Read the model definition and answer for the solid it produces. Units are mm, in the model's axes. Face numbers are marked on the shaded views. A direction names the side the tool comes from. Round coordinates to 2 decimals unless told otherwise and drop trailing zeros. Order: outer loops, then holes, each group sorted by start corner. A loop starts at its lowest first (then second) coordinate and runs counter-clockwise, first axis right, second up. Notation, with made-up numbers: (32.5, 54.5) -> (88.5, 54.5) arc R24 ccw to (88.5, 77.5) -> close; hole circle Ø10 at (48, 73.5). An arc over 180 degrees is marked (long way). One line per item, written item: value. Start each with the question number.
1. Flat-ended cylindrical pins translate along their axes: pin 1 Ø7 at (x, y) = (10, 4) entering from +Z; pin 2 Ø3 at (y, z) = (1, 85) entering from +X; pin 3 Ø1.6 at (x, y) = (0.5, 13) entering from +Z; pin 4 Ø5 at (x, z) = (8.5, -71.5) entering from -Y. Find the tip coordinate at first contact, or state that the pin passes through.
2. Section B-B (z = -38) is taken. Give the vertices of the cut face in (x, y).
3. Consider line 1 (Y direction, x = 0, z = 80); line 2 (Z direction, x = 4.75, y = -11); line 3 (Z direction, x = 9.5, y = -0.25). Determine where each line is inside the solid, lowest interval first.
4. Section A-A (z = 76) is taken. Give the vertices of the cut face in (x, y), then the cut area to 3 significant figures.
5. For the marked faces 1, 2 and 3, determine the directions among +Z, -Z, +X, -X, +Y, -Y from which every point of the face is accessible in a straight line to the end or side of a thin tool.
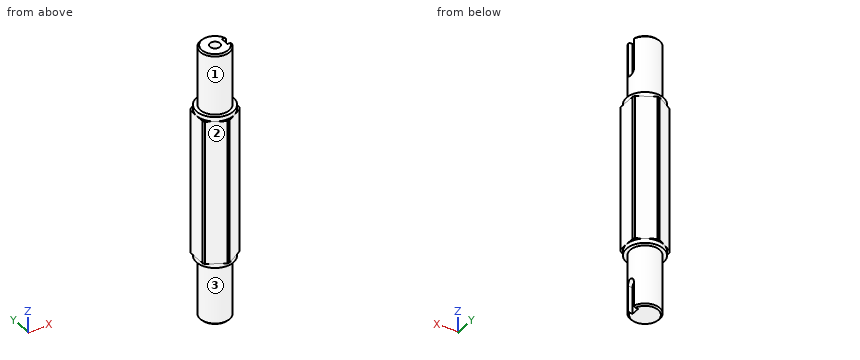
from build123d import *

# Parameters (mm, degrees)
BOSS_EXTRUDE1_DEPTH   = 49
CHAMFER1_SIZE         = 1
M8_TAPPED_HOLE1_D     = 6.8
M8_TAPPED_HOLE1_DEPTH = 19.75
M8_TAPPED_HOLE1_TIP   = 2.042926105
CUT_EXTRUDE1_START    = 10
CUT_EXTRUDE1_DEPTH    = 3.5


with BuildPart() as part:
    # Sketch1 → Boss-Extrude1 (new, symmetric)
    with BuildSketch(Plane.XY):
        with BuildLine():
            ThreePointArc((0.789917583, 13.977697601), (0, 14), (-0.789917583, 13.977697601))
            Line((-0.789917583, 13.977697601), (-11.710082417, 7.672937494))
            ThreePointArc((-11.710082417, 7.672937494), (-12.124355653, 7), (-12.5, 6.304760106))
            Line((-12.5, 6.304760106), (-12.5, -6.304760106))
            ThreePointArc((-12.5, -6.304760106), (-12.124355653, -7), (-11.710082417, -7.672937494))
            Line((-11.710082417, -7.672937494), (-0.789917583, -13.977697601))
            ThreePointArc((-0.789917583, -13.977697601), (0, -14), (0.789917583, -13.977697601))
            Line((0.789917583, -13.977697601), (11.710082417, -7.672937494))
            ThreePointArc((11.710082417, -7.672937494), (12.124355653, -7), (12.5, -6.304760106))
            Line((12.5, -6.304760106), (12.5, 6.304760106))
            ThreePointArc((12.5, 6.304760106), (12.124355653, 7), (11.710082417, 7.672937494))
            Line((11.710082417, 7.672937494), (0.789917583, 13.977697601))
        make_face()
    extrude(amount=BOSS_EXTRUDE1_DEPTH, both=True)

    # Sketch2 → Revolve1 (revolve)
    with BuildSketch(Plane(origin=(0, 0, 0), x_dir=(0, 0, -1), z_dir=(1, 0, 0)), mode=Mode.PRIVATE) as revolve1_sk:
        Polygon((-93, 0), (-93, 10), (-52, 10), (-52, 12.5), (-49, 12.5), (-49, 0), align=None)
        Polygon((52, 10), (93, 10), (93, 0), (49, 0), (49, 12.5), (52, 12.5), align=None)
    revolve(revolve1_sk.sketch.rotate(Axis((0, 0, -70.752525622), (0, 0, 1)), 90), axis=Axis((0, 0, -70.752525622), (0, 0, 1)))

    # Chamfer1
    chamfer1_edges = [part.edges().sort_by_distance(p)[0] for p in [
        (10, 0, 93),
        (10, 0, -93),
    ]]
    chamfer(chamfer1_edges, length=CHAMFER1_SIZE)

    # M8 Tapped Hole1
    with Locations(Plane.XY.offset(93)):
        with Locations((0, 0)):
            Hole(M8_TAPPED_HOLE1_D / 2, depth=M8_TAPPED_HOLE1_DEPTH)
            with Locations((0, 0, -(M8_TAPPED_HOLE1_DEPTH + M8_TAPPED_HOLE1_TIP / 2))):  # 118° drill point
                Cone(0, M8_TAPPED_HOLE1_D / 2, M8_TAPPED_HOLE1_TIP, mode=Mode.SUBTRACT)

    # Sketch4 → Cut-Extrude1 (cut)
    with BuildSketch(Plane(origin=(0, 0, 0), x_dir=(0, 0, -1), z_dir=(1, 0, 0)).offset(CUT_EXTRUDE1_START)):
        with BuildLine():
            Line((-93, -3), (-71, -3))
            ThreePointArc((-71, -3), (-68, 0), (-71, 3))
            Line((-71, 3), (-93, 3))
            ThreePointArc((-93, 3), (-96, 0), (-93, -3))
        make_face()
        with BuildLine():
            Line((93, 3), (75, 3))
            ThreePointArc((75, 3), (72, 0), (75, -3))
            Line((75, -3), (93, -3))
            ThreePointArc((93, -3), (96, 0), (93, 3))
        make_face()
    extrude(amount=-CUT_EXTRUDE1_DEPTH, mode=Mode.SUBTRACT)


solid = part.part
Answer:
1. pin 1: z = 93
1. pin 2: x = 6.5
1. pin 3: z = 52
1. pin 4: y = -8
2. outline: (-12.5, -6.3) arc R14 ccw to (-11.71, -7.67) -> (-0.79, -13.98) arc R14 ccw to (0.79, -13.98) -> (11.71, -7.67) arc R14 ccw to (12.5, -6.3) -> (12.5, 6.3) arc R14 ccw to (11.71, 7.67) -> (0.79, 13.98) arc R14 ccw to (-0.79, 13.98) -> (-11.71, 7.67) arc R14 ccw to (-12.5, 6.3) -> close
3. line 1: -10 to -3.4, 3.4 to 10
3. line 2: -52 to 52
3. line 3: -72.01 to 68.01
4. outline: (6.5, -3) -> (6.5, 3) -> (9.54, 3) arc R10 ccw (long way) to (9.54, -3) -> close; hole circle Ø6.8 at (0, 0)
4. area: 258 mm^2
5. face 1: +Z
5. face 2: +Z, -Z, -X, -Y
5. face 3: -Z
